For this review, take the finished solid that the model builds, in its own axes (mm). A direction names the side the tool comes from. Give positions to 0.01 mm unless a question says otherwise; leave off trailing zeros. Order: outer loops, then holes, each group sorted by start corner. A loop starts at its lowest first (then second) coordinate and runs counter-clockwise, first axis right, second up. Notation, with made-up numbers: (87.25, -9) - (123.25, -9) arc R19 cw to (123.25, 11) - close; hole circle Ø8 at (56.25, 32). An arc over 180 degrees is marked (long way). Answer as a JSON object with one key per item and string values. Group by question number.
from build123d import *

# Parameters (mm, degrees)
BOSS_EXTRUDE1_DEPTH             = 10.6
SKETCH2_R                       = 16.5
CUT_EXTRUDE1_DEPTH              = 0.6
SKETCH3_R                       = 11
BOSS_EXTRUDE2_DEPTH             = 2.6
SKETCH4_R                       = 3.25
CUT_EXTRUDE2_DEPTH              = 2
SKETCH5_R                       = 2.5
CUT_EXTRUDE3_DEPTH              = 11.6
FILLET1_R                       = 0.5
FILLET2_R                       = 0.5
M3X0_5_TAPPED_HOLE1_D           = 2.5
M3X0_5_TAPPED_HOLE1_DEPTH       = 10
M3X0_5_TAPPED_HOLE1_CSINK_D     = 3.5
M3X0_5_TAPPED_HOLE1_CSINK_ANGLE = 90
M3X0_5_TAPPED_HOLE1_TIP         = 0.751075774
SKETCH10_W                      = 26.901846944
SKETCH10_H                      = 2.5
CUT_EXTRUDE4_DEPTH              = 43.3
SKETCH11_W                      = 26.901846944
SKETCH11_H                      = 2.5
CUT_EXTRUDE5_DEPTH              = 43.3
FILLET3_R                       = 2


with BuildPart() as part:
    # Sketch1 → Boss-Extrude1 (new body)
    with BuildSketch(Plane(origin=(0, 0, 0), x_dir=(1, 0, 0), z_dir=(0, 1, 0))):
        Polygon((-21.15, 16.750923472), (-16.750923472, 21.15), (16.750923472, 21.15), (21.15, 16.750923472), (21.15, -16.750923472), (16.750923472, -21.15), (-16.750923472, -21.15), (-21.15, -16.750923472), align=None)
    extrude(amount=BOSS_EXTRUDE1_DEPTH)

    # Sketch2 → Cut-Extrude1 (cut)
    with BuildSketch(Plane(origin=(0, 10.6, 0), x_dir=(1, 0, 0), z_dir=(0, 1, 0))):
        Circle(SKETCH2_R)
    extrude(amount=-CUT_EXTRUDE1_DEPTH, mode=Mode.SUBTRACT)

    # Sketch3 → Boss-Extrude2 (add)
    with BuildSketch(Plane(origin=(0, 10, 0), x_dir=(1, 0, 0), z_dir=(0, 1, 0))):
        Circle(SKETCH3_R)
    extrude(amount=BOSS_EXTRUDE2_DEPTH)

    # Sketch4 → Cut-Extrude2 (cut)
    with BuildSketch(Plane(origin=(0, 12.6, 0), x_dir=(1, 0, 0), z_dir=(0, 1, 0))):
        Circle(SKETCH4_R)
    extrude(amount=-CUT_EXTRUDE2_DEPTH, mode=Mode.SUBTRACT)

    # Sketch5 → Cut-Extrude3 (cut, through all)
    with BuildSketch(Plane(origin=(0, 10.6, 0), x_dir=(1, 0, 0), z_dir=(0, 1, 0))):
        Circle(SKETCH5_R)
    extrude(amount=-CUT_EXTRUDE3_DEPTH, mode=Mode.SUBTRACT)

    # Fillet1
    fillet1_edges = [part.edges().sort_by_distance(p)[0] for p in [
        (-3.25, 12.6, 0),
    ]]
    fillet(fillet1_edges, radius=FILLET1_R)

    # Fillet2
    fillet2_edges = [part.edges().sort_by_distance(p)[0] for p in [
        (-11, 10, 0),
    ]]
    fillet(fillet2_edges, radius=FILLET2_R)

    # M3x0.5 Tapped Hole1
    with Locations(Plane(origin=(0, 10.6, 0), x_dir=(1, 0, 0), z_dir=(0, 1, 0))):
        with Locations((-15.5, 15.5), (15.5, 15.5), (15.5, -15.5), (-15.5, -15.5)):
            CounterSinkHole(M3X0_5_TAPPED_HOLE1_D / 2, M3X0_5_TAPPED_HOLE1_CSINK_D / 2, depth=M3X0_5_TAPPED_HOLE1_DEPTH, counter_sink_angle=M3X0_5_TAPPED_HOLE1_CSINK_ANGLE)
            with Locations((0, 0, -(M3X0_5_TAPPED_HOLE1_DEPTH + M3X0_5_TAPPED_HOLE1_TIP / 2))):  # 118° drill point
                Cone(0, M3X0_5_TAPPED_HOLE1_D / 2, M3X0_5_TAPPED_HOLE1_TIP, mode=Mode.SUBTRACT)

    # Sketch10 → Cut-Extrude4 (cut, through all)
    with BuildSketch(Plane.XY.offset(21.15)):
        with Locations((0, 1.25)):
            Rectangle(SKETCH10_W, SKETCH10_H)
    extrude(amount=-CUT_EXTRUDE4_DEPTH, mode=Mode.SUBTRACT)

    # Sketch11 → Cut-Extrude5 (cut, through all)
    with BuildSketch(Plane.ZY.offset(21.15)):
        with Locations((0, 1.25)):
            Rectangle(SKETCH11_W, SKETCH11_H)
    extrude(amount=-CUT_EXTRUDE5_DEPTH, mode=Mode.SUBTRACT)

    # Fillet3
    fillet3_edges = [part.edges().sort_by_distance(p)[0] for p in [
        (-21.15, 5.3, -16.750923472),
        (-16.750923472, 5.3, -21.15),
        (16.750923472, 5.3, -21.15),
        (21.15, 5.3, -16.750923472),
        (21.15, 5.3, 16.750923472),
        (16.750923472, 5.3, 21.15),
        (-16.750923472, 5.3, 21.15),
        (-21.15, 5.3, 16.750923472),
    ]]
    fillet(fillet3_edges, radius=FILLET3_R)


solid = part.part
1) Consider section A-A (y = 1.25). Give the number of separate pieces and of enclosed holes in the cut face, plus the area to 3 significant figures.
2) For pin 1 (3 mm diameter, centred on x = -15.5, z = 15.5, fed in from -Y); pin 2 (12.5 mm diameter, centred on x = -7.5, z = -1, fed in from -Y); pin 3 (1.5 mm diameter, centred on x = 15.5, z = 15.5, fed in from +Y); pin 4 (0.8 mm diameter, centred on y = 1, z = -18, fed in from -X), all flat-tipped, find the tip position at first contact; note any pin that passes through.
3) For faces 4 (the face through (19, 5.2, 18.9)), 5 (the face through (-2.579, 11.36, 1.978)), 6 (the face through (-17, 1, 13.451)), list the 3-axis set-ups (+Z, -Z, +X, -X, +Y, -Y) from which the entire face can be reached by the end or side of a thin tool; tool diameter is ignored.
4) Mouldability with a two-part tool opening along Z and no side actions: class faces 1 (the face through (2, 10.6, 2)), 2 (the face through (18.9, 5.2, -19)), 3 (the face through (-13.451, 1, -17)) as released by +Z, released by -Z, zero draft, split by the parting line, or undercut.
5) Consider section D-D (y = 8.25). Give the boundary of the cut face in (x, z).
6) Consider section C-C (z = 0). Give the boundary of the cut face in (x, y).
7) For line 1 (Z direction, x = -15.5, y = 6.25); line 2 (X direction, y = 10.5, z = -5.5); line 3 (Z direction, x = 0, y = 11.45), list the stretches that pass through material, from the lowest coordinate up.
8) Consider section B-B (x = 0). Give the boundary of the cut face in (y, z).
Result set:
{
 "1": {"separate pieces": "4", "enclosed holes": "4", "area": "178 mm2"},
 "2": {"pin 1": "stops at y = 0", "pin 2": "stops at y = 2.5", "pin 3": "stops at y = 0.3", "pin 4": "stops at x = -20.3"},
 "3": {"face 4": "+Z, +X, +Y, -Y", "face 5": "+Y", "face 6": "+X, -X, -Y"},
 "4": {"face 1": "undercut", "face 2": "released by -Z", "face 3": "zero draft"},
 "5": {"outline": "(-21.15, -15.92) arc R2 ccw to (-20.56, -17.34) - (-17.34, -20.56) arc R2 ccw to (-15.92, -21.15) - (15.92, -21.15) arc R2 ccw to (17.34, -20.56) - (20.56, -17.34) arc R2 ccw to (21.15, -15.92) - (21.15, 15.92) arc R2 ccw to (20.56, 17.34) - (17.34, 20.56) arc R2 ccw to (15.92, 21.15) - (-15.92, 21.15) arc R2 ccw to (-17.34, 20.56) - (-20.56, 17.34) arc R2 ccw to (-21.15, 15.92) - close; hole circle Ø2.5 at (-15.5, -15.5); hole circle Ø2.5 at (-15.5, 15.5); hole circle Ø5 at (0, 0); hole circle Ø2.5 at (15.5, -15.5); hole circle Ø2.5 at (15.5, 15.5)"},
 "6": {"outline": "(-21.15, 2.5) - (-2.5, 2.5) - (-2.5, 10.6) - (-3.25, 10.6) - (-3.25, 12.1) arc R0.5 ccw to (-3.75, 12.6) - (-11, 12.6) - (-11, 10.5) arc R0.5 cw to (-11.5, 10) - (-16.5, 10) - (-16.5, 10.6) - (-21.15, 10.6) - close; (2.5, 2.5) - (21.15, 2.5) - (21.15, 10.6) - (16.5, 10.6) - (16.5, 10) - (11.5, 10) arc R0.5 cw to (11, 10.5) - (11, 12.6) - (3.75, 12.6) arc R0.5 ccw to (3.25, 12.1) - (3.25, 10.6) - (2.5, 10.6) - close"},
 "7": {"line 1": "z = -21.15 to -16.75, -14.25 to 14.25, 16.75 to 21.15", "line 2": "x = -21.15 to -15.56, -9.53 to 9.53, 15.56 to 21.15", "line 3": "z = -11 to -3.25, 3.25 to 11"},
 "8": {"outline": "(2.5, -21.15) - (10.6, -21.15) - (10.6, -16.5) - (10, -16.5) - (10, -11.5) arc R0.5 cw to (10.5, -11) - (12.6, -11) - (12.6, -3.75) arc R0.5 ccw to (12.1, -3.25) - (10.6, -3.25) - (10.6, -2.5) - (2.5, -2.5) - close; (2.5, 2.5) - (10.6, 2.5) - (10.6, 3.25) - (12.1, 3.25) arc R0.5 ccw to (12.6, 3.75) - (12.6, 11) - (10.5, 11) arc R0.5 cw to (10, 11.5) - (10, 16.5) - (10.6, 16.5) - (10.6, 21.15) - (2.5, 21.15) - close"}
}
